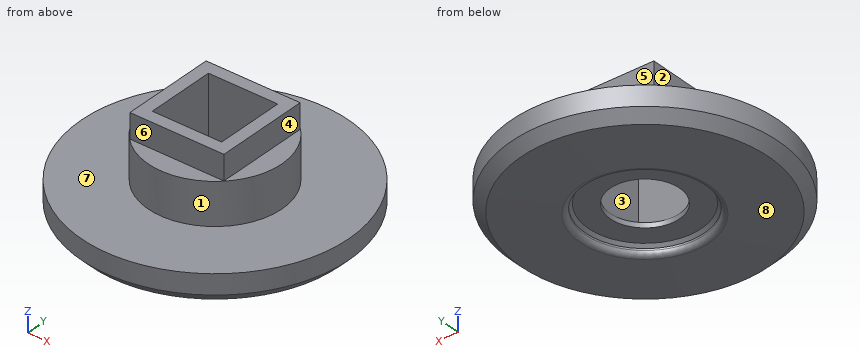
from build123d import *

# Parameters (mm, degrees)
CYLINDER_R                 = 3.5
CYLINDER_DEPTH             = 13
BOX001_W                   = 7
BOX001_H                   = 7
BOX001_DEPTH               = 10.5
BOX_W                      = 9.5
BOX_H                      = 9.5
BOX_DEPTH                  = 9
CHAMFER_SIZE               = 0.3
FILLET_R                   = 0.5
CHAMFER001_SIZE            = 1
CHAMFER001_PLACEMENT_ANGLE = 180


with BuildPart() as cilindro:
    # Cylinder → Cylinder (new body)
    with BuildSketch(Plane.XY.offset(-5)):
        Circle(CYLINDER_R)
    extrude(amount=CYLINDER_DEPTH)


with BuildPart() as cubo001:
    # Box001 → Box001 (new body)
    with BuildSketch(Plane(origin=(-3.5, -3.5, -4.5), x_dir=(1, 0, 0), z_dir=(0, 0, 1))):
        with Locations((3.5, 3.5)):
            Rectangle(BOX001_W, BOX001_H)
    extrude(amount=BOX001_DEPTH)


with BuildPart() as cubo:
    # Box → Box (new body)
    with BuildSketch(Plane(origin=(-4.75, -4.75, -2.5), x_dir=(1, 0, 0), z_dir=(0, 0, 1))):
        with Locations((4.75, 4.75)):
            Rectangle(BOX_W, BOX_H)
    extrude(amount=BOX_DEPTH)


with BuildPart() as chamfer001:
    # Sketch → Revolution (revolve)
    with BuildSketch(Plane.XZ):
        Polygon((0, 0), (0, 6.5), (6, 6.5), (6, 7.5), (13.5, 7.238094), (13.5, 4.238094), (6.75, 4.238094), (6.75, 0), align=None)
    revolve(axis=Axis((0, 0, 0), (0, 0, 1)))

    # Fusion: union Cubo
    add(cubo.part)

    # Cut: cut Cubo001
    add(cubo001.part, mode=Mode.SUBTRACT)

    # Cut001: cut Cilindro
    add(cilindro.part, mode=Mode.SUBTRACT)

    # Chamfer
    chamfer_edges = [chamfer001.edges().sort_by_distance(p)[0] for p in [
        (5.678908, 1.936492, 6.5),
    ]]
    chamfer(chamfer_edges, length=CHAMFER_SIZE)

    # Fillet
    fillet_edges = [chamfer001.edges().sort_by_distance(p)[0] for p in [
        (-6, 0, 7.5),
    ]]
    fillet(fillet_edges, radius=FILLET_R)

    # Chamfer001
    chamfer001_edges = [chamfer001.edges().sort_by_distance(p)[0] for p in [
        (-13.5, 0, 7.238094),
    ]]
    chamfer(chamfer001_edges, length=CHAMFER001_SIZE)


with BuildPart() as chamfer001_1:
    # Chamfer001 placement: moved
    add(chamfer001.part.rotate(Axis((0, 0, 0), (1, 0, 0)), CHAMFER001_PLACEMENT_ANGLE))


solid = chamfer001_1.part
Read the model definition and answer for the solid it produces. Units are mm, in the model's axes. Face numbers are marked on the shaded views. A direction names the side the tool comes from. Give positions to 0.01 mm unless a question says otherwise; leave off trailing zeros. Write each loop counter-clockwise with the first axis right and the second up, starting at its lowest first coordinate (ties: lowest second). Pieces come first, ordered by that corner, then holes. Notation, with made-up numbers: (-2.5, 0) - (18.5, 0) arc R30 cw to (18.5, 24) - close; hole circle Ø7 at (84, 37.25). An arc over 180 degrees is marked (long way). Answer in a Markdown table with one row per item. Add a question column.
Item 1: A tool of negligible diameter and unlimited length cuts with its end or side. For the marked faces 4, 5, 6, 7 and 8, from which of +Z, -Z, +X, -X, +Y, -Y can it reach the whole face along a straight path? Write none if from no direction.
Item 2: Section B-B, the plane z = -4.75 is taken. Write down the section's boundary in (x, y), and give its area (3 significant figures).
Item 3: Find the intervals of material crossed by L1, parallel to Y at x = 0, z = -6.1; L2, parallel to X at y = 0, z = -6.85; L3, parallel to X at y = 2.25, z = -5, in increasing order.
Item 4: Flat-ended cylindrical pins translate along their axes: P1, Ø1, axis at x = -8, y = 0.5, coming from the -Z side; P2, Ø4, axis at x = 9.5, z = -3.5, coming from the +Y side; P3, Ø1, axis at x = 2, y = 2, coming from the +Z side; P4, Ø3.5, axis at y = -1, z = -0.5, coming from the +X side. Find the tip coordinate at first contact, or state that the pin passes through.
Item 5: Determine the mould class of the marked faces 1, 2 and 3 for opening direction Y: pulls with the +Y half, pulls with the -Y half, needs draft (parallel to the pull), parting line crosses it, or undercut.
Item 6: Section A-A, the plane z = 0.75 is taken. Write down the section's boundary in (x, y), and give its area (4 significant figures).
Recorded:
| question | item | result |
|---|---|---|
| 1 | face 4 | +Z, +X, +Y, -Y |
| 1 | face 5 | +Z, +X, -X, +Y |
| 1 | face 6 | +Z, +X, -X, -Y |
| 1 | face 7 | +Z |
| 1 | face 8 | -Z |
| 2 | outline | circle Ø27 at (0, 0); hole (-3.5, -3.5) - (3.5, -3.5) - (3.5, 3.5) - (-3.5, 3.5) - close |
| 2 | area | 524 mm2 |
| 3 | L1 | y = -13.5 to -3.5, 3.5 to 13.5 |
| 3 | L2 | x = -12.91 to -6, 6 to 12.91 |
| 3 | L3 | x = -13.31 to -3.5, 3.5 to 13.31 |
| 4 | P1 | stops at z = -7.45 |
| 4 | P2 | stops at y = 11.13 |
| 4 | P3 | passes through |
| 4 | P4 | stops at x = 6.75 |
| 5 | face 1 | parting line crosses it |
| 5 | face 2 | needs draft |
| 5 | face 3 | undercut |
| 6 | outline | (-4.75, -4.75) - (4.75, -4.75) - (4.75, 4.75) - (-4.75, 4.75) - close; hole (-3.5, -3.5) - (3.5, -3.5) - (3.5, 3.5) - (-3.5, 3.5) - close |
| 6 | area | 41.25 mm2 |
